Autodesk Inventor part; units mm, degrees
ref_plane "YZ Plane" through (0, 0, 0) normal (1, 0, 0) x (0, 1, 0)
ref_plane "XZ Plane" through (0, 0, 0) normal (0, 1, 0) x (-1, 0, 0)
ref_plane "XY Plane" through (0, 0, 0) normal (0, 0, 1) x (1, 0, 0)
sketch "Sketch1" plane through (0, 0, 0) normal (0, 0, 1) x (1, 0, 0)
  line L0 (0, 0) -> (-11.15, 0)
  line L1 (-11.15, 0) -> (-11.15, 26)
  line L2 (-11.15, 26) -> (-8, 26)
  line L3 (-8, 26) -> (-8, 33)
  line L4 (-8, 33) -> (-6, 33)
  line L5 (-6, 33) -> (-6, 39)
  line L6 (-6, 39) -> (-8, 39)
  line L7 (-8, 39) -> (-8, 42.7)
  line L8 (-8, 42.7) -> (0, 42.7)
  line L9 (0, 42.7) -> (0, 0)
  dimension "d0" = 6
  dimension "d2" = 8
  dimension "d3" = 11.15
  dimension "d4" = 26
  dimension "d5" = 42.7
  dimension "d6" = 3.7
  dimension "d7" = 6
revolve "Revolution1" add sketch "Sketch1" angle 360 about axis through (0, 42.7, 0) along (0, -1, 0)
sketch "Sketch2" plane through (0, 0, 0) normal (0, 0, 1) x (1, 0, 0)
  line L0 (11.15, 26) -> (11.15, 0)
  line L1 (11.15, 0) -> (-11.15, 0)
  line L2 (-11.15, 0) -> (-11.15, 26)
  line L3 (-11.15, 26) -> (-8, 26)
  line L4 (-8, 26) -> (-8, 33)
  line L5 (-8, 33) -> (-6, 33)
  line L6 (-6, 33) -> (-6, 39)
  line L7 (-6, 39) -> (-8, 39)
  line L8 (-8, 39) -> (-8, 42.7)
  line L9 (-8, 42.7) -> (8, 42.7)
  line L10 (8, 42.7) -> (8, 39)
  line L11 (8, 39) -> (6, 39)
  line L12 (6, 39) -> (6, 33)
  line L13 (6, 33) -> (8, 33)
  line L14 (8, 33) -> (8, 26)
  line L15 (8, 26) -> (11.15, 26)
  line L16 (-11.15, 1) -> (-6, 1)
  line L17 (-6, 1) -> (-6, 2.5)
  line L18 (-6, 2.5) -> (-11.15, 2.5)
  line L19 (-11.15, 2.5) -> (-11.15, 1)
  line L20 (0, -8.54) -> (0, 51.24)
  point P0 (0, 0)
  dimension "d9" = 6
  dimension "d10" = 1.5
  dimension "d11" = 1
revolve "Revolution2" cut sketch "Sketch2" angle 360 about axis through (0, -10, 0) along (0, 1, 0) contours L2 L18 L17 L16
pattern_linear "Rectangular Pattern1" count 12 spacing 2.5 along (0, 1, 0) of "Revolution2"
sketch "Sketch3" plane through (0, 0, 0) normal (0, -1, 0) x (1, 0, 0)
  circle A0 centre (0, 0) radius 11.15
  circle A1 centre (0, 0) radius 1.4
  dimension "d16" = 2.8
extrude "Extrusion1" add sketch "Sketch3" along normal blind 2.1 contours A1
sketch "Sketch4" plane through (0, -2.1, 0) normal (0, -1, 0) x (1, 0, 0)
  circle A0 centre (0, 0) radius 1.4
  line L0 (-4.5, 8) -> (15.5, 8)
  line L1 (15.5, 8) -> (15.5, -8)
  line L2 (15.5, -8) -> (-4.5, -8)
  line L3 (-4.5, -8) -> (-4.5, 8)
  point P0 (-4.5, 0)
  dimension "d20" = 4.5
  dimension "d21" = 16
  dimension "d22" = 20
extrude "Extrusion2" add sketch "Sketch4" along normal blind 11.5 contours A0 | L0 L1 L2 L3
sketch "Sketch5" plane through (-4.5, -2.1, 8) normal (0, 0, 1) x (1, 0, 0)
  line L0 (0, 0) -> (0, -11.5)
  line L1 (20, -11.5) -> (0, -11.5)
  line L2 (20, 0) -> (20, -11.5)
  circle A0 centre (11.5, -7.5) radius 3
  line L3 (11.5, -6.75) -> (20, -6.75)
  line L4 (20, -6.75) -> (20, -8.25)
  line L5 (20, -8.25) -> (11.5, -8.25)
  line L6 (11.5, -8.25) -> (11.5, -6.75)
  point P0 (4.5, 2.1)
  dimension "d25" = 4
  dimension "d26" = 6
  dimension "d27" = 1.5
  dimension "d28" = 11.5
extrude "Extrusion3" cut sketch "Sketch5" against normal through all
sketch "Sketch6" plane through (0, -13.6, 0) normal (0, -1, 0) x (1, 0, 0)
  circle A0 centre (0, 0) radius 2.5
  dimension "d32" = 5
extrude "Extrusion4" add sketch "Sketch6" along normal blind 1.5
fillet "Fillet1" radius 1 14 edges at (5.5, -2.1, 8) (15.5, -5.475, 8) (15.5, -5.475, -8) (15.5, -2.1, 0) (5.5, -2.1, -8) (-4.5, -7.85, -8) (-4.5, -2.1, 0) (-4.5, -7.85, 8) (-4.5, -13.6, 0) (5.5, -13.6, -8) (15.5, -11.975, -8) (15.5, -13.6, 0) (15.5, -11.975, 8) (5.5, -13.6, 8)
sketch "Sketch7" plane through (0, -15.1, 0) normal (0, -1, 0) x (1, 0, 0)
  circle A0 centre (0, 0) radius 2.5
  line L0 (2.0207, 3.5) -> (4.0415, 0)
  line L1 (4.0415, 0) -> (2.0207, -3.5)
  line L2 (2.0207, -3.5) -> (-2.0207, -3.5)
  line L3 (-2.0207, -3.5) -> (-4.0415, 0)
  line L4 (-4.0415, 0) -> (-2.0207, 3.5)
  line L5 (-2.0207, 3.5) -> (2.0207, 3.5)
  dimension "d36" = 7
extrude "Extrusion5" add sketch "Sketch7" along normal blind 3 contours A0 | L0 L1 L2 L3 L4 L5
sketch "Sketch8" plane through (0, 0, 0) normal (0, 0, 1) x (1, 0, 0)
  line L0 (6, 2.5) -> (6, 1)
  line L1 (6, 1) -> (11.15, 1)
  line L2 (11.15, 1) -> (11.15, 0)
  line L3 (11.15, 0) -> (1.4, 0)
  line L4 (1.4, 0) -> (1.4, -2.1)
  line L5 (1.4, -2.1) -> (14.5, -2.1)
  arc A0 (15.5, -3.1) -> (14.5, -2.1) centre (14.5, -3.1) ccw
  line L6 (15.5, -3.1) -> (15.5, -8.85)
  line L7 (15.5, -8.85) -> (9.9047, -8.85)
  arc A1 (9.9047, -8.85) -> (9.9047, -10.35) centre (7, -9.6) ccw
  line L8 (9.9047, -10.35) -> (15.5, -10.35)
  line L9 (15.5, -10.35) -> (15.5, -12.6)
  arc A2 (14.5, -13.6) -> (15.5, -12.6) centre (14.5, -12.6) ccw
  line L10 (14.5, -13.6) -> (2.5, -13.6)
  line L11 (2.5, -13.6) -> (2.5, -15.1)
  line L12 (2.5, -15.1) -> (4.0415, -15.1)
  line L13 (4.0415, -15.1) -> (4.0415, -18.1)
  line L14 (4.0415, -18.1) -> (-4.0415, -18.1)
  line L15 (-4.0415, -18.1) -> (-4.0415, -15.1)
  line L16 (-4.0415, -15.1) -> (-2.5, -15.1)
  line L17 (-2.5, -15.1) -> (-2.5, -13.6)
  line L18 (-2.5, -13.6) -> (-3.5, -13.6)
  arc A3 (-4.5, -12.6) -> (-3.5, -13.6) centre (-3.5, -12.6) ccw
  line L19 (-4.5, -12.6) -> (-4.5, -3.1)
  arc A4 (-3.5, -2.1) -> (-4.5, -3.1) centre (-3.5, -3.1) ccw
  line L20 (-3.5, -2.1) -> (-1.4, -2.1)
  line L21 (-1.4, -2.1) -> (-1.4, 0)
  line L22 (-1.4, 0) -> (-11.15, 0)
  line L23 (-11.15, 0) -> (-11.15, 1)
  line L24 (-11.15, 1) -> (-6, 1)
  line L25 (-6, 1) -> (-6, 2.5)
  line L26 (-6, 2.5) -> (-11.15, 2.5)
  line L27 (-11.15, 2.5) -> (-11.15, 3.5)
  line L28 (-11.15, 3.5) -> (-6, 3.5)
  line L29 (-6, 3.5) -> (-6, 5)
  line L30 (-6, 5) -> (-11.15, 5)
  line L31 (-11.15, 5) -> (-11.15, 6)
  line L32 (-11.15, 6) -> (-6, 6)
  line L33 (-6, 6) -> (-6, 7.5)
  line L34 (-6, 7.5) -> (-11.15, 7.5)
  line L35 (-11.15, 7.5) -> (-11.15, 8.5)
  line L36 (-11.15, 8.5) -> (-6, 8.5)
  line L37 (-6, 8.5) -> (-6, 10)
  line L38 (-6, 10) -> (-11.15, 10)
  line L39 (-11.15, 10) -> (-11.15, 11)
  line L40 (-11.15, 11) -> (-6, 11)
  line L41 (-6, 11) -> (-6, 12.5)
  line L42 (-6, 12.5) -> (-11.15, 12.5)
  line L43 (-11.15, 12.5) -> (-11.15, 13.5)
  line L44 (-11.15, 13.5) -> (-6, 13.5)
  line L45 (-6, 13.5) -> (-6, 15)
  line L46 (-6, 15) -> (-11.15, 15)
  line L47 (-11.15, 15) -> (-11.15, 16)
  line L48 (-11.15, 16) -> (-6, 16)
  line L49 (-6, 16) -> (-6, 17.5)
  line L50 (-6, 17.5) -> (-11.15, 17.5)
  line L51 (-11.15, 17.5) -> (-11.15, 18.5)
  line L52 (-11.15, 18.5) -> (-6, 18.5)
  line L53 (-6, 18.5) -> (-6, 20)
  line L54 (-6, 20) -> (-11.15, 20)
  line L55 (-11.15, 20) -> (-11.15, 21)
  line L56 (-11.15, 21) -> (-6, 21)
  line L57 (-6, 21) -> (-6, 22.5)
  line L58 (-6, 22.5) -> (-11.15, 22.5)
  line L59 (-11.15, 22.5) -> (-11.15, 23.5)
  line L60 (-11.15, 23.5) -> (-6, 23.5)
  line L61 (-6, 23.5) -> (-6, 25)
  line L62 (-6, 25) -> (-11.15, 25)
  line L63 (-11.15, 25) -> (-11.15, 26)
  line L64 (-11.15, 26) -> (-6, 26)
  line L65 (-6, 26) -> (-6, 27.5)
  line L66 (-6, 27.5) -> (-8, 27.5)
  line L67 (-8, 27.5) -> (-8, 28.5)
  line L68 (-8, 28.5) -> (-6, 28.5)
  line L69 (-6, 28.5) -> (-6, 30)
  line L70 (-6, 30) -> (-8, 30)
  line L71 (-8, 30) -> (-8, 33)
  line L72 (-8, 33) -> (-6, 33)
  line L73 (-6, 33) -> (-6, 39)
  line L74 (-6, 39) -> (-8, 39)
  line L75 (-8, 39) -> (-8, 42.7)
  line L76 (-8, 42.7) -> (8, 42.7)
  line L77 (8, 42.7) -> (8, 39)
  line L78 (8, 39) -> (6, 39)
  line L79 (6, 39) -> (6, 33)
  line L80 (6, 33) -> (8, 33)
  line L81 (8, 33) -> (8, 30)
  line L82 (8, 30) -> (6, 30)
  line L83 (6, 30) -> (6, 28.5)
  line L84 (6, 28.5) -> (8, 28.5)
  line L85 (8, 28.5) -> (8, 27.5)
  line L86 (8, 27.5) -> (6, 27.5)
  line L87 (6, 27.5) -> (6, 26)
  line L88 (6, 26) -> (11.15, 26)
  line L89 (11.15, 26) -> (11.15, 25)
  line L90 (11.15, 25) -> (6, 25)
  line L91 (6, 25) -> (6, 23.5)
  line L92 (6, 23.5) -> (11.15, 23.5)
  line L93 (11.15, 23.5) -> (11.15, 22.5)
  line L94 (11.15, 22.5) -> (6, 22.5)
  line L95 (6, 22.5) -> (6, 21)
  line L96 (6, 21) -> (11.15, 21)
  line L97 (11.15, 21) -> (11.15, 20)
  line L98 (11.15, 20) -> (6, 20)
  line L99 (6, 20) -> (6, 18.5)
  line L100 (6, 18.5) -> (11.15, 18.5)
  line L101 (11.15, 18.5) -> (11.15, 17.5)
  line L102 (11.15, 17.5) -> (6, 17.5)
  line L103 (6, 17.5) -> (6, 16)
  line L104 (6, 16) -> (11.15, 16)
  line L105 (11.15, 16) -> (11.15, 15)
  line L106 (11.15, 15) -> (6, 15)
  line L107 (6, 15) -> (6, 13.5)
  line L108 (6, 13.5) -> (11.15, 13.5)
  line L109 (11.15, 13.5) -> (11.15, 12.5)
  line L110 (11.15, 12.5) -> (6, 12.5)
  line L111 (6, 12.5) -> (6, 11)
  line L112 (6, 11) -> (11.15, 11)
  line L113 (11.15, 11) -> (11.15, 10)
  line L114 (11.15, 10) -> (6, 10)
  line L115 (6, 10) -> (6, 8.5)
  line L116 (6, 8.5) -> (11.15, 8.5)
  line L117 (11.15, 8.5) -> (11.15, 7.5)
  line L118 (11.15, 7.5) -> (6, 7.5)
  line L119 (6, 7.5) -> (6, 6)
  line L120 (6, 6) -> (11.15, 6)
  line L121 (11.15, 6) -> (11.15, 5)
  line L122 (11.15, 5) -> (6, 5)
  line L123 (6, 5) -> (6, 3.5)
  line L124 (6, 3.5) -> (11.15, 3.5)
  line L125 (11.15, 3.5) -> (11.15, 2.5)
  line L126 (11.15, 2.5) -> (6, 2.5)
  line L127 (0, -18.1) -> (0, -20.1)
  line L128 (0, -20.1) -> (-0.5, -20.1)
  line L129 (-0.5, -20.1) -> (-1.9004, -18.1)
  point P0 (0, 0)
  dimension "d39" = 125
  dimension "d41" = 0.5
  dimension "d42" = 2
revolve "Revolution3" add sketch "Sketch8" angle 360 about axis through (0, -18.1, 0) along (0, -1, 0) contours L127 L128 L129 L14
properties part number "E3Dv6"
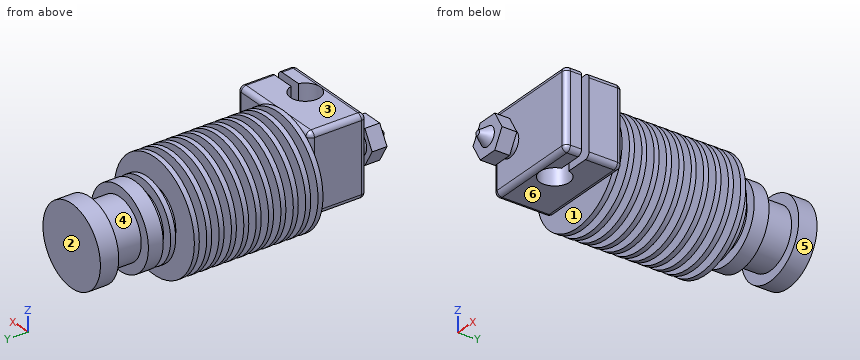
Read the model definition and answer for the solid it produces. Units are mm, in the model's axes. Face numbers are marked on the shaded views. A direction names the side the tool comes from. Coordinates: 2 decimals unless noted, no trailing zeros. Loops run counter-clockwise (first coordinate to the right, second up) from the corner with the lowest first, then second, coordinate; pieces in that order, holes last. Notation, with made-up numbers: (-40, 89) - (-1, 89) arc R21 cw to (-1, 111) - close; hole circle Ø9 at (70.5, 56.5). An arc over 180 degrees is marked (long way). Answer in a Markdown table with one row per item.
1. Find section C-C, the plane y = -9.6. Write down the section's boundary in (x, z).
Conclusion:
| item | result |
|---|---|
| outline | (-4.5, -7) arc R1 ccw to (-3.5, -8) - (4, -8) - (4, 8) - (-3.5, 8) arc R1 ccw to (-4.5, 7) - close |
2. Find section A-A, the plane y = -16. Write down the section's boundary in (x, z).
Conclusion:
| item | result |
|---|---|
| outline | (-4.04, 0) - (-2.02, -3.5) - (2.02, -3.5) - (4.04, 0) - (2.02, 3.5) - (-2.02, 3.5) - close |
3. Find section B-B, the plane x = 7. Count the separate pieces of the cut face and the enclosed holes in it, then the cut area to 3 significant figures.
Conclusion:
| item | result |
|---|---|
| separate pieces | 16 |
| enclosed holes | 0 |
| area | 338 mm² |
4. Which of the six approach directions +Z, -Z, +X, -X, +Y, -Y give full straight-line access (tool end or side, diameter ignored) to the marked faces 4, 5 and 6?
Conclusion:
| item | result |
|---|---|
| face 4 | none |
| face 5 | +Y |
| face 6 | -Z, +X, -X, -Y |
5. Determine the mould class of the marked faces 1, 2 and 3 for opening direction Y: +Y half, -Y half, draft (parallel to the pull), parting line (faces both ways), or undercut.
Conclusion:
| item | result |
|---|---|
| face 1 | undercut |
| face 2 | +Y half |
| face 3 | draft |
6. Straight lines are drawn through the part: line 1 (Y direction, x = 1.75, z = -5.5); line 2 (Y direction, x = 12, z = -4); line 3 (X direction, y = -9.6, z = -3.75). For each, find the intervals that lie inside material, in ascending order.
Conclusion:
| item | result |
|---|---|
| line 1 | y = -13.6 to -2.1, 0 to 42.7 |
| line 2 | y = -13.6 to -10.35, -8.85 to -2.1 |
| line 3 | x = -4.5 to 4 |
7. Given pin 1 (6.5 mm diameter, centred on x = -1, z = 5, fed in from -Y); pin 2 (6 mm diameter, centred on y = 36.5, z = 1.5, fed in from +X); pin 3 (3 mm diameter, centred on x = 11.5, y = -12.5, fed in from -Z), each flat-ended and moving along its own axis, determine where each tip first touches the part or whether it passes through.
Conclusion:
| item | result |
|---|---|
| pin 1 | stops at y = -18.17 |
| pin 2 | stops at x = 8 |
| pin 3 | stops at z = -8 |
